from build123d import *

# Parameters (mm, degrees)
F0_W     = 100
F0_H     = 100
F1_DEPTH = 100
F2_R     = 10
F3_DEPTH = 20
F4_R     = 10


with BuildPart() as f1:
    # F0 (on Top) → F1 (new body)
    with BuildSketch(Plane.XY):
        with Locations((50, 50)):
            Rectangle(F0_W, F0_H)
    extrude(amount=-F1_DEPTH)

    # F2 (on face) → F3 (join)
    with BuildSketch(Plane.XY):
        with Locations((50, 50)):
            Circle(F2_R)
    extrude(amount=F3_DEPTH)

    # F4
    f4_edges = [f1.edges().sort_by_distance(p)[0] for p in [
        (0, 0, -50),
        (100, 0, -50),
        (50, 0, 0),
        (50, 0, -100),
        (100, 50, 0),
        (100, 100, -50),
        (50, 100, 0),
        (0, 50, 0),
        (50, 100, -100),
        (0, 100, -50),
        (0, 50, -100),
        (100, 50, -100),
    ]]
    fillet(f4_edges, radius=F4_R)


solid = f1.part
The model under review builds one solid part; all positions refer to its coordinate system, in mm. A direction names the side the tool comes from. Coordinates: 2 decimals unless noted, no trailing zeros. Loops run counter-clockwise (first coordinate to the right, second up) from the corner with the lowest first, then second, coordinate; pieces in that order, holes last. Notation, with made-up numbers: M 47,53.25 L 69,53.25 A26 cw 69,88.25 Z; hole C 58.25,-21 d9. An arc over 180 degrees is marked long. Put each result on its own line as item: value. Start each with the question number.
Q1. Add section C-C (z = -8). Write out the cut boundary in (x, y), and give its area (3 significant figures).
Q2. For faces 1 (the cylindrical face through (2.85, 3.01, -50.56)), 2 (the flat face through (58, 59, 0)), list the 3-axis set-ups (+Z, -Z, +X, -X, +Y, -Y) from which the entire face can be reached by the end or side of a thin tool; tool diameter is ignored.
Q3. Add section A-A (x = 50). Write out the cut boundary in (y, z).
Q4. Wall thickness on line 1 (Z direction, x = 43, y = 66); line 2 (Z direction, x = 62, y = 95); line 3 (Y direction, x = 7, z = -28): over which ranges is each line inside the solid? List them lowest first.
Q5. Add section B-B (y = 25). Write out the cut boundary in (x, z), and give its area (3 significant figures).
Q6. Clearance check with a flat-ended pin moving along its axis: pin 1 (1.5 mm diameter, centred on x = 22, y = 56.5, fed in from +Z). State where the tip first meets the part, or that it passes through.
Answers:
1. outline: M 0.2,10 A9.8 ccw 10,0.2 L 90,0.2 A9.8 ccw 99.8,10 L 99.8,90 A9.8 ccw 90,99.8 L 10,99.8 A9.8 ccw 0.2,90 Z
1. area: 9,840 mm^2
2. face 1: +Z, -Z, -X, -Y
2. face 2: +Z
3. outline: M 0,-90 A10 ccw 10,-100 L 90,-100 A10 ccw 100,-90 L 100,-10 A10 ccw 90,0 L 60,0 L 60,20 L 40,20 L 40,0 L 10,0 A10 ccw 0,-10 Z
4. line 1: z = -100 to 0
4. line 2: z = -98.66 to -1.34
4. line 3: y = 0.46 to 99.54
5. outline: M 0,-90 A10 ccw 10,-100 L 90,-100 A10 ccw 100,-90 L 100,-10 A10 ccw 90,0 L 10,0 A10 ccw 0,-10 Z
5. area: 9,910 mm^2
6. pin 1: stops at z = 0
